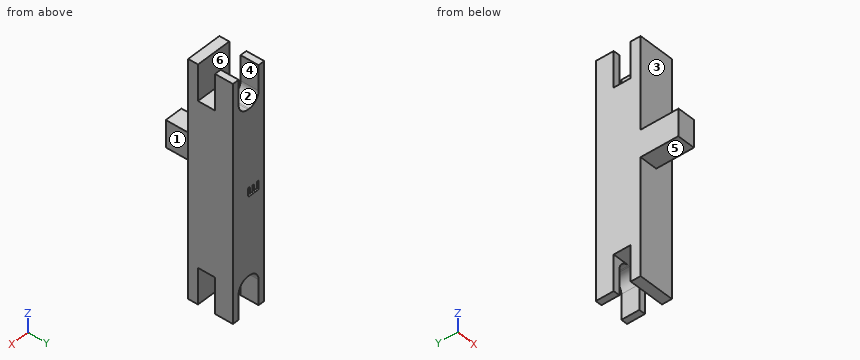
```python
from build123d import *

# Parameters (mm, degrees)
SKETCH2_W            = 10.16
SKETCH2_H            = 66.675
BOSS_EXTRUDE1_DEPTH  = 12.7
SKETCH3_W            = 5.08
SKETCH3_H            = 6.35
SKETCH3_H_2          = 1.27
BOSS_EXTRUDE2_DEPTH  = 12.7
CUT_EXTRUDE1_DEPTH   = 10.16
FILLET2_R            = 3.048
FILLET2_OF_MIRROR1_R = 3.048
CUT_EXTRUDE4_DEPTH   = 69.629958655
CUT_EXTRUDE5_DEPTH   = 0.508


with BuildPart() as part:
    # Sketch2 → Boss-Extrude1 (new body)
    with BuildSketch(Plane(origin=(0, 0, 0), x_dir=(1, 0, 0), z_dir=(0, 1, 0))):
        with Locations((5.08, 33.3375)):
            Rectangle(SKETCH2_W, SKETCH2_H)
    extrude(amount=BOSS_EXTRUDE1_DEPTH)

    # Sketch3 → Boss-Extrude2 (add)
    with BuildSketch(Plane.XZ):
        with Locations((2.54, -29.21)):
            Rectangle(SKETCH3_W, SKETCH3_H)
        with Locations((2.54, -33.02)):
            Rectangle(SKETCH3_W, SKETCH3_H_2)
    extrude(amount=BOSS_EXTRUDE2_DEPTH)

    # Sketch4 → Cut-Extrude1 (cut)
    with BuildSketch(Plane.XY):
        Polygon((0, 7.62), (1.8415, 7.62), (1.8415, 12.7), (8.3185, 12.7), (8.3185, 7.62), (10.16, 7.62), (10.16, 2.794), (0, 2.794), align=None)
    cut_extrude1 = extrude(amount=-CUT_EXTRUDE1_DEPTH, mode=Mode.SUBTRACT)

    # Fillet2
    fillet2_edges = [part.edges().sort_by_distance(p)[0] for p in [
        (1.8415, 10.16, -10.16),
        (8.3185, 10.16, -10.16),
    ]]
    fillet(fillet2_edges, radius=FILLET2_R)

    # Mirror1: Cut-Extrude1 across plane
    add(cut_extrude1.mirror(Plane.XY.offset(-33.3375)), mode=Mode.SUBTRACT)

    # Fillet2 of Mirror1
    fillet2_of_mirror1_edges = [part.edges().sort_by_distance(p)[0] for p in [
        (1.8415, 10.16, -56.515),
        (8.3185, 10.16, -56.515),
    ]]
    fillet(fillet2_of_mirror1_edges, radius=FILLET2_OF_MIRROR1_R)

    # Sketch5 → Cut-Extrude4 (cut, through all)
    with BuildSketch(Plane.ZY):
        with BuildLine():
            Line((-66.675, -12.7), (0, -12.7))
            ThreePointArc((0, -12.7), (-33.3375, -10.668), (-66.675, -12.7))
        make_face()
    extrude(amount=-CUT_EXTRUDE4_DEPTH, mode=Mode.SUBTRACT)

    # Sketch6 → Cut-Extrude5 (cut)
    with BuildSketch(Plane(origin=(0, 12.7, 0), x_dir=(1, 0, 0), z_dir=(0, 1, 0))):
        with BuildLine():
            Line((4.68525, 32.318945312), (4.68525, 33.8625))
            Line((4.68525, 33.8625), (3.854, 33.8625))
            Line((3.854, 33.8625), (3.854, 32.441308594))
            add(Edge.make_bspline(
                [(3.854, 32.441308594), (3.85306664, 32.416646376), (3.85131467, 32.370353963), (3.838922285, 32.305553354), (3.816176667, 32.250750116), (3.784435917, 32.206165385), (3.744958065, 32.171924109), (3.699953428, 32.146753392), (3.648447348, 32.132038096), (3.612331739, 32.130427428), (3.593550781, 32.129589844)],
                knots=[0, 0, 0, 0, 1.285293232, 2.412569968, 3.418386025, 4.354403319, 5.23810445, 6.120527863, 7.022630715, 8, 8, 8, 8], degree=3))
            add(Edge.make_bspline(
                [(3.593550781, 32.129589844), (3.574749437, 32.130386162), (3.538594625, 32.131917475), (3.487376628, 32.147184911), (3.441067547, 32.170468115), (3.400708139, 32.204601131), (3.368216057, 32.249315164), (3.344656766, 32.304313536), (3.331515928, 32.36960597), (3.329873624, 32.416410782), (3.329, 32.441308594)],
                knots=[0, 0, 0, 0, 0.970712631, 1.866671451, 2.742370236, 3.637940775, 4.57451605, 5.578136324, 6.711690039, 8, 8, 8, 8], degree=3))
            Line((3.329, 32.441308594), (3.329, 33.8625))
            Line((3.329, 33.8625), (2.3665, 33.8625))
            Line((2.3665, 33.8625), (2.3665, 32.265625))
            add(Edge.make_bspline(
                [(2.3665, 32.265625), (2.3655501, 32.240286731), (2.363764391, 32.192653494), (2.351476637, 32.125480995), (2.328025391, 32.068668897), (2.296333649, 32.021515895), (2.256316564, 31.985404245), (2.210438968, 31.958523559), (2.157768886, 31.943480459), (2.120952669, 31.941339483), (2.101949219, 31.940234375)],
                knots=[0, 0, 0, 0, 1.282115211, 2.410239491, 3.433544999, 4.370413449, 5.259840111, 6.137762651, 7.038767785, 8, 8, 8, 8], degree=3))
            add(Edge.make_bspline(
                [(2.101949219, 31.940234375), (2.083387815, 31.94130204), (2.047657894, 31.943357251), (1.99647574, 31.958830307), (1.951565967, 31.985590419), (1.911713519, 32.021521306), (1.879780454, 32.068510842), (1.857617463, 32.125745925), (1.843908263, 32.192526909), (1.842335714, 32.24025854), (1.8415, 32.265625)],
                knots=[0, 0, 0, 0, 0.94634305, 1.821670557, 2.697075277, 3.594139625, 4.539053153, 5.56674892, 6.706875008, 8, 8, 8, 8], degree=3))
            Line((1.8415, 32.265625), (1.8415, 34.116796875))
            add(Edge.make_bspline(
                [(1.8415, 34.116796875), (1.842466239, 34.150170648), (1.844264303, 34.212275576), (1.862680376, 34.298270852), (1.892787961, 34.369951249), (1.937907595, 34.427362709), (1.998445006, 34.469083716), (2.072427477, 34.499358574), (2.16166782, 34.515384672), (2.225621192, 34.517576552), (2.259859375, 34.51875)],
                knots=[0, 0, 0, 0, 1.189944925, 2.214356848, 3.121275872, 3.943259729, 4.783004917, 5.7166381, 6.777575619, 8, 8, 8, 8], degree=3))
            Line((2.259859375, 34.51875), (4.791890625, 34.51875))
            add(Edge.make_bspline(
                [(4.791890625, 34.51875), (4.81537587, 34.518197938), (4.859971724, 34.517149635), (4.923783566, 34.510060607), (4.980566831, 34.496281007), (5.031331248, 34.478007659), (5.075573059, 34.45409369), (5.113745466, 34.424163537), (5.144476669, 34.387304712), (5.169662361, 34.344901006), (5.187624682, 34.296110527), (5.20161385, 34.241903477), (5.208592234, 34.181233065), (5.209681005, 34.138913293), (5.21025, 34.116796875)],
                knots=[0, 0, 0, 0, 1.25760687, 2.388054849, 3.429687073, 4.379296607, 5.269270079, 6.111463577, 6.959732887, 7.823909447, 8.739278143, 9.733531743, 10.815538057, 12, 12, 12, 12], degree=3))
            Line((5.21025, 34.116796875), (5.21025, 32.318945312))
            add(Edge.make_bspline(
                [(5.21025, 32.318945312), (5.209294138, 32.293380123), (5.207496341, 32.245296836), (5.195306163, 32.177659161), (5.1719504, 32.120727753), (5.140037158, 32.074132036), (5.100434178, 32.038946704), (5.055076035, 32.013331032), (5.003864768, 31.998014319), (4.967678458, 31.99642215), (4.949117187, 31.995605469)],
                knots=[0, 0, 0, 0, 1.303543407, 2.451718649, 3.482873774, 4.417375591, 5.305837532, 6.158811619, 7.05558772, 8, 8, 8, 8], degree=3))
            add(Edge.make_bspline(
                [(4.949117187, 31.995605469), (4.930090551, 31.996389194), (4.893210146, 31.997908334), (4.841038001, 32.013538139), (4.794569462, 32.03849449), (4.754855556, 32.074202728), (4.722711227, 32.120560462), (4.700417628, 32.177846336), (4.68793119, 32.245265971), (4.686180707, 32.293369409), (4.68525, 32.318945312)],
                knots=[0, 0, 0, 0, 0.961524532, 1.863777426, 2.731626687, 3.61454628, 4.543218546, 5.563575511, 6.704588277, 8, 8, 8, 8], degree=3))
        make_face()
    extrude(amount=-CUT_EXTRUDE5_DEPTH, mode=Mode.SUBTRACT)


solid = part.part
```
For this review, take the finished solid that the model builds, in its own axes (mm). Face numbers are marked on the shaded views. A direction names the side the tool comes from. Round coordinates to 2 decimals unless told otherwise and drop trailing zeros. Loops run counter-clockwise (first coordinate to the right, second up) from the corner with the lowest first, then second, coordinate; pieces in that order, holes last.
(1) Tool access review of the marked faces 4, 5 and 6: name each direction out of +Z, -Z, +X, -X, +Y, -Y from which nothing blocks a thin tool from reaching the whole face with its end or side.
Returned:
face 4: +Z, +Y
face 5: -Z, +X, -X, -Y
face 6: +Z, +X, -X
(2) We need section A-A (x = 9.25). Give the boundary of the cut face in (y, z) (3 decimals).
Returned:
outline: (0, -66.675) - (2.794, -66.675) - (2.794, -56.515) - (7.62, -56.515) - (7.62, -66.675) - (12.7, -66.675) - (12.7, 0) - (7.62, 0) - (7.62, -10.16) - (2.794, -10.16) - (2.794, 0) - (0, 0) - close
(3) Wall thickness on line 1 along Y through (x, z) = (2, -10); line 2 along X through (y, z) = (10.5, -60.5); line 3 along Y through (x, z) = (9.5, -25.5): over which ranges is each line inside the solid? List them lowest first.
Returned:
line 1: y = 0 to 2.79, 7.62 to 12.7
line 2: x = 0 to 1.84, 8.32 to 10.16
line 3: y = 0 to 12.7
(4) Mouldability with a two-part tool opening along X and no side actions: class the marked faces 1, 2 and 3 as released by +X, released by -X, zero draft, split by the parting line, or undercut.
Returned:
face 1: released by +X
face 2: undercut
face 3: zero draft
(5) We need section D-D (z = -41). Give the boundary of the cut face in (x, y).
Returned:
outline: (0, 0) - (10.16, 0) - (10.16, 12.7) - (0, 12.7) - close
(6) We need section B-B (z = -58). Give the boundary of the cut face in (x, y).
Returned:
outline: (0, 0) - (10.16, 0) - (10.16, 2.79) - (0, 2.79) - close; (0, 7.62) - (2.27, 7.62) - (2.27, 12.7) - (0, 12.7) - close; (7.89, 7.62) - (10.16, 7.62) - (10.16, 12.7) - (7.89, 12.7) - close
(7) Clearance check with flat-ended pins moving along their axes: P1, Ø2.5, axis at x = 8.5, z = -62.5, coming from the -Y side; P2, Ø2.5, axis at y = -6.5, z = -30, coming from the +X side; P3, Ø5.5, axis at y = 11, z = -64, coming from the -X side; P4, Ø1.5, axis at x = 6, y = 9.5, coming from the +Z side. State where each tip first meets the part, or that it passes through.
Returned:
P1: stops at y = 0
P2: stops at x = 5.08
P3: stops at x = 0
P4: stops at z = -9.78
